Geometry: see drawing. Coordinates: mm, zero at the bounding-box minimum. Coordinates: 2 decimals unless noted, no trailing zeros. Loops run counter-clockwise (first coordinate to the right, second up) from the corner with the lowest first, then second, coordinate; pieces in that order, holes last. Notation, with made-up numbers: (6, 9) - (15, 9) arc R17 ccw to (15, 21) - close; hole circle Ø2 at (50, 44). An arc over 180 degrees is marked (long way). Use one line per item in the form item = value.
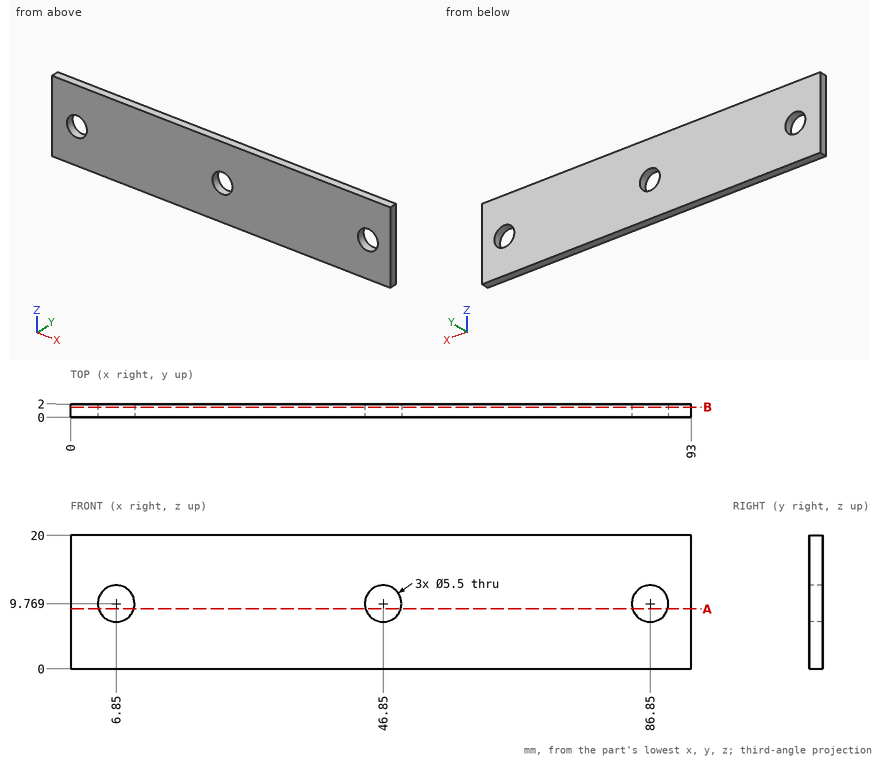
Q1. First-contact query: P1, Ø3.5, axis at x = 46.85, z = 9.77, coming from the -Y side. Flat tip, straight axial feed; report the tip coordinate or a pass-through.
Check values:
P1 = through
Q2. Cut plane A-A, the plane z = 9. Return loops of the section in (x, y), then the cut area to 3 significant figures.
Check values:
outline = (0, 0) - (4.21, 0) - (4.21, 2) - (0, 2) - close; (9.49, 0) - (44.21, 0) - (44.21, 2) - (9.49, 2) - close; (49.49, 0) - (84.21, 0) - (84.21, 2) - (49.49, 2) - close; (89.49, 0) - (93, 0) - (93, 2) - (89.49, 2) - close
area = 154 mm²
Q3. Ray query, line 1 along X through (y, z) = (0.5, 9.5); line 2 along X through (y, z) = (1.05, 8.25). Return the intervals inside material, ascending. Write a range as [from, to].
Check values:
line_1 = [0, 4.11], [9.59, 44.11], [49.59, 84.11], [89.59, 93]
line_2 = [0, 4.56], [9.14, 44.56], [49.14, 84.56], [89.14, 93]
Q4. Cut plane B-B, the plane y = 1.55. Return loops of the section in (x, z), then the cut area to 3 significant figures.
Check values:
outline = (0, 0) - (93, 0) - (93, 20) - (0, 20) - close; hole circle Ø5.5 at (6.85, 9.77); hole circle Ø5.5 at (46.85, 9.77); hole circle Ø5.5 at (86.85, 9.77)
area = 1,790 mm²
